Part model, mm, in its own coordinate system. Face numbers are marked on the shaded views. A direction names the side the tool comes from. Coordinates: 2 decimals unless noted, no trailing zeros. Write each loop counter-clockwise with the first axis right and the second up, starting at its lowest first coordinate (ties: lowest second). Pieces come first, ordered by that corner, then holes. Notation, with made-up numbers: (-9.5, 75.5) - (11.5, 75.5) arc R26 ccw to (11.5, 105.5) - close; hole circle Ø11 at (-38, -15). An arc over 180 degrees is marked (long way). Use a Markdown table: item, result.
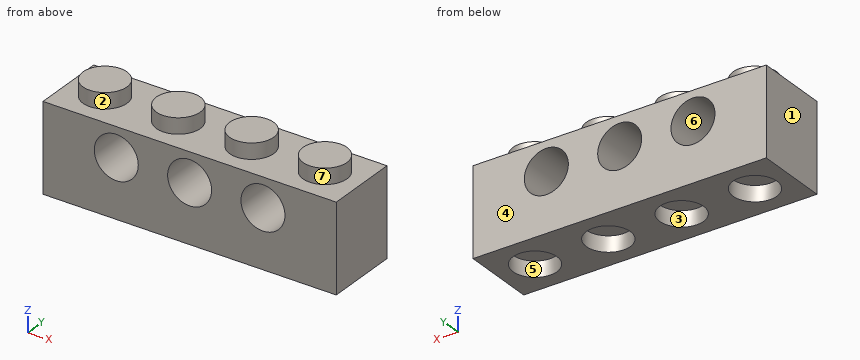
```python
from build123d import *

# Parameters (mm, degrees)
F1_DEPTH  = 8
F3_W      = 8
F3_H      = 8
F3_R      = 2.4
F4_DEPTH  = 1.7
F5_R      = 2.4
F6_DEPTH  = 1.7
F11_R     = 2.4
F12_DEPTH = 25.4


with BuildPart() as f1:
    # F0 (on Front) → F1 (new body)
    with BuildSketch(Plane.XZ):
        Polygon((-2.4, 9.6), (-4, 9.6), (-4, 0), (4, 0), (4, 9.6), (2.4, 9.6), (2.4, 11.3), (-2.4, 11.3), align=None)
    extrude(amount=F1_DEPTH)

    # F3 (on plane+point) → F4 (cut, through all)
    with BuildSketch(Plane.XY.offset(11.3)):
        with Locations((0, -4)):
            Rectangle(F3_W, F3_H)
        with Locations((0, -4)):
            Circle(F3_R, mode=Mode.SUBTRACT)
    extrude(amount=-F4_DEPTH, mode=Mode.SUBTRACT)

    # F5 (on Top) → F6 (cut)
    with BuildSketch(Plane.XY):
        with Locations((0, -4)):
            Circle(F5_R)
    extrude(amount=F6_DEPTH, mode=Mode.SUBTRACT)

    # F8: F1 across plane


with BuildPart() as f1_1:
    add(f1.part)
    add(f1.part.mirror(Plane.YZ.offset(4)))

    # F10: F1 across plane


with BuildPart() as f1_2:
    add(f1_1.part)
    add(f1_1.part.mirror(Plane.YZ.offset(12)))

    # F11 (on Front) → F12 (cut)
    with BuildSketch(Plane.XZ):
        with Locations((19.999, 6.4008)):
            Circle(F11_R)
        with Locations((11.998, 6.4008)):
            Circle(F11_R)
        with Locations((3.997, 6.4008)):
            Circle(F11_R)
    extrude(amount=F12_DEPTH, mode=Mode.SUBTRACT)


solid = f1_2.part
```
Item 1: Which spindle directions (+Z, -Z, +X, -X, +Y, -Y) get a long thin tool onto all of the face, cutting with end or side? Do the marked faces 1, 2 and 3. Say none if no direction does.
From the geometry:
| item | result |
|---|---|
| face 1 | +Z, -Z, -X, +Y, -Y |
| face 2 | +Z |
| face 3 | -Z |
Item 2: Band-saw the part on B-B, the plane z = 6.75. Give the cut face in (x, y).
From the geometry:
| item | result |
|---|---|
| outline | (-4, -8) - (1.62, -8) - (1.62, 0) - (-4, 0) - close; (6.37, -8) - (9.62, -8) - (9.62, 0) - (6.37, 0) - close; (14.37, -8) - (17.62, -8) - (17.62, 0) - (14.37, 0) - close; (22.37, -8) - (28, -8) - (28, 0) - (22.37, 0) - close |
Item 3: Band-saw the part on C-C, the plane x = 0. Give the cut face in (y, z), then the cut area to 3 significant figures.
From the geometry:
| item | result |
|---|---|
| outline | (-8, 0) - (-6.4, 0) - (-6.4, 1.7) - (-1.6, 1.7) - (-1.6, 0) - (0, 0) - (0, 9.6) - (-1.6, 9.6) - (-1.6, 11.3) - (-6.4, 11.3) - (-6.4, 9.6) - (-8, 9.6) - close |
| area | 76.8 mm^2 |
Item 4: Two-plate mould, pull along Y, no slides. Class the marked faces 4, 5, 6 and 7: pulls with the +Y half, pulls with the -Y half, needs draft (parallel to the pull), parting line crosses it, or undercut.
From the geometry:
| item | result |
|---|---|
| face 4 | pulls with the +Y half |
| face 5 | undercut |
| face 6 | needs draft |
| face 7 | parting line crosses it |
Item 5: Drop flat-ended pins along their axis: P1, Ø1, axis at x = 9.5, y = -1, coming from the +Z side; P2, Ø4, axis at x = 8, y = -4, coming from the -Z side; P3, Ø4, axis at x = 20, z = 6.4, coming from the +Y side. Give the stop position or say it passes through.
From the geometry:
| item | result |
|---|---|
| P1 | z = 9.6 |
| P2 | z = 1.7 |
| P3 | through |
Item 6: Band-saw the part on A-A, the plane y = -7.25. Give the cut face in (x, z).
From the geometry:
| item | result |
|---|---|
| outline | (-4, 0) - (28, 0) - (28, 9.6) - (-4, 9.6) - close; hole circle Ø4.8 at (4, 6.4); hole circle Ø4.8 at (12, 6.4); hole circle Ø4.8 at (20, 6.4) |
Item 7: Drill centre lines: probe 1 along Y at (x, z) = (0, 1.3); probe 2 along X at (y, z) = (-2.5, 0.5); probe 3 along X at (y, z) = (-0.75, 8.25). Where is each one in solid material? Low to high.
From the geometry:
| item | result |
|---|---|
| probe 1 | -8 to -6.4, -1.6 to 0 |
| probe 2 | -4 to -1.87, 1.87 to 6.13, 9.87 to 14.13, 17.87 to 22.13, 25.87 to 28 |
| probe 3 | -4 to 2.47, 5.53 to 10.47, 13.53 to 18.47, 21.53 to 28 |
